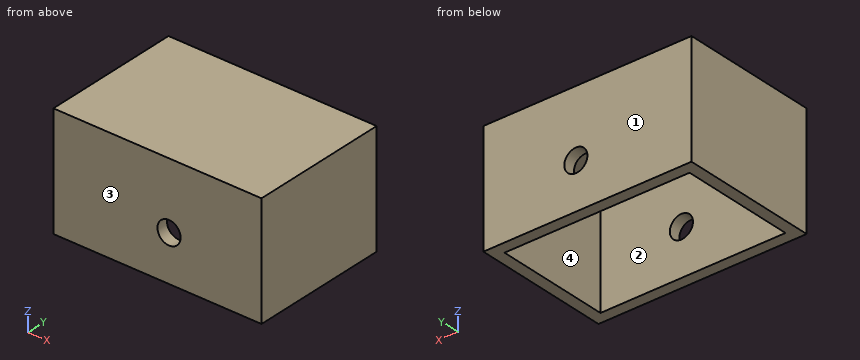
```python
from build123d import *

# Parameters (mm, degrees)
F0_W     = 114.3
F0_H     = 62.237151
F1_DEPTH = 38.1
F2_T     = -6.35
F3_R     = 6.35
F4_DEPTH = 76.201


with BuildPart() as f1:
    # F0 (on Front) → F1 (new body, symmetric)
    with BuildSketch(Plane.XZ):
        with Locations((57.15, 31.118575)):
            Rectangle(F0_W, F0_H)
    extrude(amount=F1_DEPTH, both=True)

    # F2
    f2_openings = [f1.faces().sort_by_distance(p)[0] for p in [
        (57.15, 0, 0),
    ]]
    offset(amount=F2_T, openings=f2_openings)

    # F3 (on face) → F4 (cut, through all)
    with BuildSketch(Plane.XZ.offset(38.1)):
        with Locations((63.5, 25.4)):
            Circle(F3_R)
    extrude(amount=-F4_DEPTH, mode=Mode.SUBTRACT)


solid = f1.part
```
Verification items for the finished model (mm, model axes). Face numbers are marked on the shaded views. Give positions to 0.01 mm unless a question says otherwise; leave off trailing zeros. Order: outer loops, then holes, each group sorted by start corner. A loop starts at its lowest first (then second) coordinate and runs counter-clockwise, first axis right, second up. Notation, with made-up numbers: (54.25, 53) -> (78.25, 53) arc R37 ccw to (78.25, 90) -> close; hole circle Ø5 at (9.5, -15). An arc over 180 degrees is marked (long way). Use a Markdown table: item, result.
1) Material ranges on probe 1 along Y at (x, z) = (18, 21.5); probe 2 along X at (y, z) = (-5.5, 16.5), recorded low to high.
Results:
| item | result |
|---|---|
| probe 1 | -38.1 to -31.75, 31.75 to 38.1 |
| probe 2 | 0 to 6.35, 107.95 to 114.3 |
2) Section check B-B, the plane z = 25.4. Record the boundary of the cut face in (x, y), then the cut area to 3 significant figures.
Results:
| item | result |
|---|---|
| outline | (0, -38.1) -> (57.15, -38.1) -> (57.15, -31.75) -> (6.35, -31.75) -> (6.35, 31.75) -> (57.15, 31.75) -> (57.15, 38.1) -> (0, 38.1) -> close; (69.85, -38.1) -> (114.3, -38.1) -> (114.3, 38.1) -> (69.85, 38.1) -> (69.85, 31.75) -> (107.95, 31.75) -> (107.95, -31.75) -> (69.85, -31.75) -> close |
| area | 2,100 mm² |
3) Section check A-A, the plane x = 63.5. Record the boundary of the cut face in (y, z), then the cut area to 3 significant figures.
Results:
| item | result |
|---|---|
| outline | (-38.1, 0) -> (-31.75, 0) -> (-31.75, 19.05) -> (-38.1, 19.05) -> close; (-38.1, 31.75) -> (-31.75, 31.75) -> (-31.75, 55.89) -> (31.75, 55.89) -> (31.75, 31.75) -> (38.1, 31.75) -> (38.1, 62.24) -> (-38.1, 62.24) -> close; (31.75, 0) -> (38.1, 0) -> (38.1, 19.05) -> (31.75, 19.05) -> close |
| area | 1,030 mm² |
4) Section check D-D, the plane z = 7. Record the boundary of the cut face in (x, y), then the cut area to 3 significant figures.
Results:
| item | result |
|---|---|
| outline | (0, -38.1) -> (114.3, -38.1) -> (114.3, 38.1) -> (0, 38.1) -> close; hole (6.35, -31.75) -> (107.95, -31.75) -> (107.95, 31.75) -> (6.35, 31.75) -> close |
| area | 2,260 mm² |
5) Section check C-C, the plane y = 33. Record the boundary of the cut face in (x, z).
Results:
| item | result |
|---|---|
| outline | (0, 0) -> (114.3, 0) -> (114.3, 62.24) -> (0, 62.24) -> close; hole circle Ø12.7 at (63.5, 25.4) |
6) Mould release check, pull along Y, two halves, no side actions. Record for the marked faces 1, 2, 3 and 4: pulls with the +Y half, pulls with the -Y half, needs draft (parallel to the pull), parting line crosses it, or undercut.
Results:
| item | result |
|---|---|
| face 1 | pulls with the +Y half |
| face 2 | undercut |
| face 3 | pulls with the -Y half |
| face 4 | undercut |
7) Depth check by flat-ended pin: pin 1 Ø19 at (x, y) = (71, -5.5) entering from -Z. Enter the tip coordinate at first touch or a pass-through.
Results:
| item | result |
|---|---|
| pin 1 | z = 55.89 |
